Autodesk Fusion 360 part; units mm, degrees
sketch "Sketch1" plane through (0, 0, 0) normal (0, 0, 1) x (1, 0, 0)
  line L0 (15, 0) -> (65, 0)
  line L1 (65, 30) -> (15, 30)
  arc A0 (15, 30) -> (0, 15) centre (15, 15) ccw
  arc A1 (0, 15) -> (15, 0) centre (15, 15) ccw
  arc A2 (80, 15) -> (65, 30) centre (65, 15) ccw
  arc A3 (65, 0) -> (80, 15) centre (65, 15) ccw
  line L2 (15, 15) -> (65, 15) construction
  line L3 (15, 15) -> (15, 27.5) construction
  line L4 (65, 15) -> (65, 27.5) construction
  line L5 (15, 27.5) -> (40, 27.5) construction
  circle A4 centre (15, 27.5) radius 1.5
  circle A5 centre (40, 27.5) radius 1.5
  circle A6 centre (65, 27.5) radius 1.5
  circle A7 centre (15, 2.5) radius 1.5
  circle A8 centre (40, 2.5) radius 1.5
  circle A9 centre (65, 2.5) radius 1.5
  point P0 (80, 0)
  point P1 (0, 30)
  dimension "d1" = 80
  dimension "d2" = 30
  dimension "d3" = 15
  dimension "d4" = 15
  dimension "d5" = 15
  dimension "d6" = 15
  dimension "d7" = 12.5
  dimension "d8" = 12.5
  dimension "d9" = 25
  dimension "d11" = 3
  dimension "d12" = 3
  dimension "d13" = 3
extrude "Extrude1" add sketch "Sketch1" along normal blind 16
shell "Shell1" thickness 2 removed faces 1 at (23.6999, 18.8266, 16)
hole "Hole1" at (65, 27.5, 0) at (40, 27.5, 0) at (15, 27.5, 0) at (15, 2.5, 0) at (40, 2.5, 0) at (65, 2.5, 0) direction (0, 0, -1) diameter 4 depth 1 tip angle 180 countersink diameter 4.4 countersink angle 90
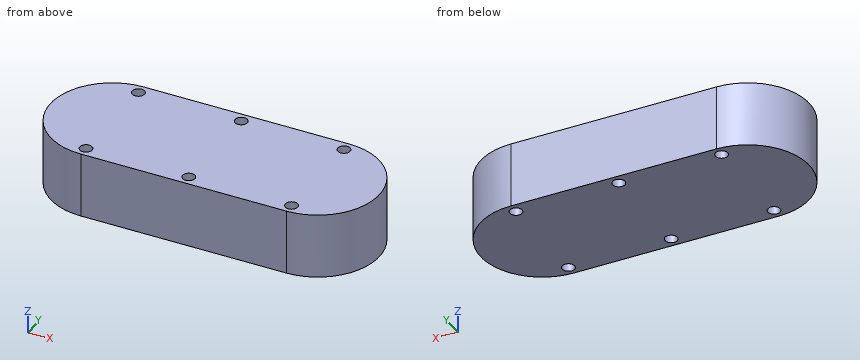
Check sheet for the modelled part. Datum: model origin and axes. Units: mm. Give positions to 0.01 mm unless a question says otherwise; leave off trailing zeros. Write each loop counter-clockwise with the first axis right and the second up, starting at its lowest first coordinate (ties: lowest second). Pieces come first, ordered by that corner, then holes. Notation, with made-up numbers: (0, -22) -> (21, -22) arc R18 ccw to (21, -5) -> close; hole circle Ø4 at (75, 72). An arc over 180 degrees is marked (long way). Use CSV: the item, a comma, the result in double quotes. Start each with the question number.
Q1. Cross-section at D-D on x = 8. Enter the section's corners in (y, z), and give its area (3 significant figures).
Q2. Depth check by flat-ended pin: P1, Ø3, axis at y = 13, z = 13, coming from the -X side; P2, Ø5, axis at y = 5.5, z = 3.5, coming from the -X side; P3, Ø1.5, axis at y = 6.5, z = 7, coming from the +X side. Enter the tip coordinate at first touch or a pass-through.
Q3. Cross-section at B-B on z = 6. Enter the section's corners in (x, y), and give its area (3 significant figures).
Q4. Cross-section at C-C on y = 27.5. Enter the section's corners in (x, z), and give its area (3 significant figures).
Q5. Scan lines: line 1 along Y through (x, z) = (65, 12.25); line 2 along Y through (x, z) = (39, 10); line 3 along Y through (x, z) = (6.5, 8). Record each from-to range of solid material in increasing order.
Q6. Cross-section at A-A on x = 40. Enter the section's corners in (y, z).
Working result:
1,outline,"(1.73, 0) -> (28.27, 0) -> (28.27, 16) -> (1.73, 16) -> close"
1,area,"425 mm^2"
2,P1,"stops at x = 0.01"
2,P2,"stops at x = 1.73"
2,P3,"stops at x = 77.84"
3,outline,"(15, 0) -> (65, 0) arc R15 ccw to (65, 30) -> (15, 30) arc R15 ccw to start; hole circle Ø3 at (15, 2.5); hole circle Ø3 at (15, 27.5); hole circle Ø3 at (40, 2.5); hole circle Ø3 at (40, 27.5); hole circle Ø3 at (65, 2.5); hole circle Ø3 at (65, 27.5)"
3,area,"2,160 mm^2"
4,outline,"(6.71, 0) -> (13.5, 0) -> (13.5, 16) -> (6.71, 16) -> close; (16.5, 0) -> (38.5, 0) -> (38.5, 16) -> (16.5, 16) -> close; (41.5, 0) -> (63.5, 0) -> (63.5, 16) -> (41.5, 16) -> close; (66.5, 0) -> (73.29, 0) -> (73.29, 16) -> (66.5, 16) -> close"
4,area,"921 mm^2"
5,line 1,"y = 0 to 1, 4 to 26, 29 to 30"
5,line 2,"y = 0 to 1.38, 3.62 to 26.38, 28.62 to 30"
5,line 3,"y = 2.64 to 27.36"
6,outline,"(0, 0) -> (1, 0) -> (1, 16) -> (0, 16) -> close; (4, 0) -> (26, 0) -> (26, 16) -> (4, 16) -> close; (29, 0) -> (30, 0) -> (30, 16) -> (29, 16) -> close"
